The drawing under review shows one solid part. Ordinate dimensions are in mm from its lowest x, y, z. Round coordinates to 2 decimals unless told otherwise and drop trailing zeros. Write each loop counter-clockwise with the first axis right and the second up, starting at its lowest first coordinate (ties: lowest second). Pieces come first, ordered by that corner, then holes. Notation, with made-up numbers: M 76.5,-15.5 L 125.5,-15.5 A23 cw 125.5,18.5 Z; hole C -9.75,-24.75 d3. An arc over 180 degrees is marked long. Write item = value, one per line. Start each with the question number.
Item 1: For pin 1 Ø3 at (x, z) = (3, 3.5) entering from +Y; pin 2 Ø2 at (y, z) = (3, 4.5) entering from -X, all flat-tipped, find the tip position at first contact; note any pin that passes through.
Item 2: Take a section at A-A, the plane x = 1.95. Give the boundary of the cut face in (y, z).
Item 3: To check wall thickness, follow line 1 along Z through (x, y) = (0.65, 3.45) (1 decimal); line 2 along Y through (x, z) = (2.6, 2) (1 decimal); line 3 along Y through (x, z) = (3.75, 3.7) (1 decimal). State the ranges of each line that lie inside material, in increasing order.
Item 4: The part is to be moulded in two halves that separate along Z. For the marked faces 1, 2 and 3, say which applies: +Z half, -Z half, draft (parallel to the pull), parting line (faces both ways), or undercut.
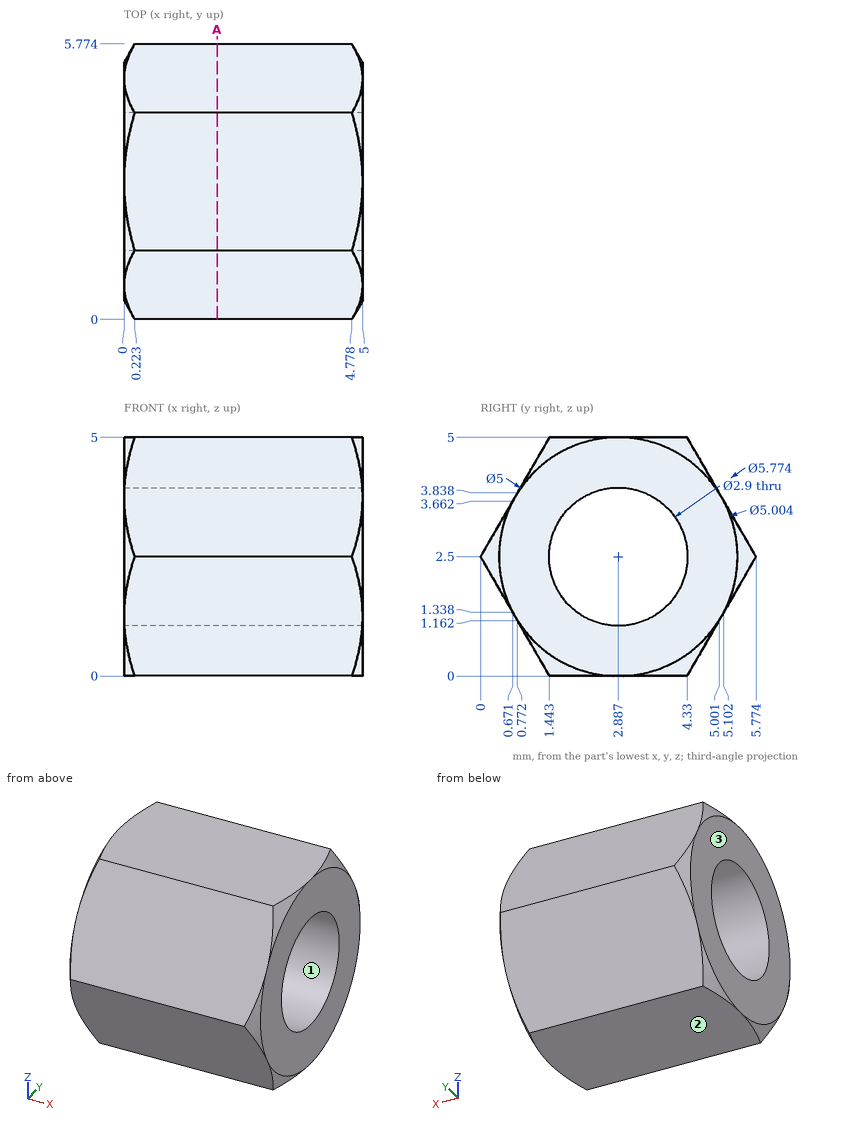
Response values:
q1.pin_1 = 5.77
q1.pin_2 = 0
q2.outline = M 0,2.5 L 1.44,0 L 4.33,0 L 5.77,2.5 L 4.33,5 L 1.44,5 Z; hole C 2.89,2.5 d2.9
q3.line_1 = 0 to 1.2, 3.8 to 5
q3.line_2 = 0.3 to 1.5, 4.2 to 5.5
q3.line_3 = 0.7 to 2.1, 3.7 to 5.1
q4.face_1 = undercut
q4.face_2 = -Z half
q4.face_3 = draft
